Job drawing, mm, ordinate dimensions from the low corner. One solid piece. A direction names the side the tool comes from. Round coordinates to 2 decimals unless told otherwise and drop trailing zeros. Loops run counter-clockwise (first coordinate to the right, second up) from the corner with the lowest first, then second, coordinate; pieces in that order, holes last.
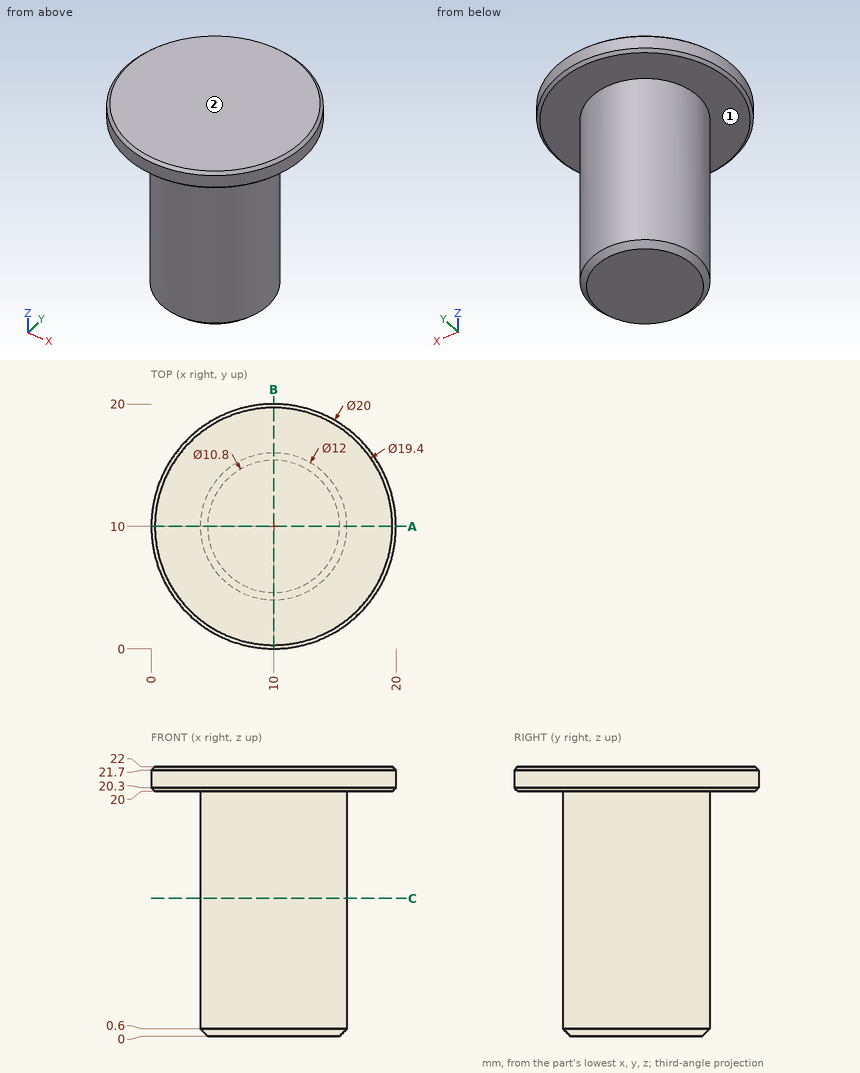
Item 1: Cut at C-C, the plane z = 11.25. Give the cut face in (x, y).
Answers follow:
outline: circle Ø12 at (10, 10)
Item 2: 3-axis set-ups, long thin cutter, end or side, ignore diameter. For the marked faces 1 and 2: which of +Z, -Z, +X, -X, +Y, -Y reach the whole face in a straight line?
Answers follow:
face 1: -Z
face 2: +Z, +X, -X, +Y, -Y
Item 3: Flat gauge pins, fed straight in: P1, Ø2, axis at y = 12, z = 12, coming from the -X side; P2, Ø6, axis at x = 17, z = 18.5, coming from the -Y side; P3, Ø2, axis at y = 10.5, z = 14, coming from the -X side. Where does each tip first touch, or does it go through?
Answers follow:
P1: stops at x = 4.08
P2: stops at y = 1.12
P3: stops at x = 4
Item 4: Probe line 1 (Z direction, x = 2, y = 8); line 2 (Y direction, x = 9.5, z = 21.25); line 3 (X direction, y = 10.5, z = 10.75). List the from-to ranges inside material, lowest first.
Answers follow:
line 1: z = 20 to 22
line 2: y = 0.01 to 19.99
line 3: x = 4.02 to 15.98
Item 5: Cut at A-A, the plane y = 10. Give the cut face in (x, z), plus the area to 3 significant figures.
Answers follow:
outline: (0, 20.3) - (0.3, 20) - (4, 20) - (4, 0.6) - (4.6, 0) - (15.4, 0) - (16, 0.6) - (16, 20) - (19.7, 20) - (20, 20.3) - (20, 21.7) - (19.7, 22) - (0.3, 22) - (0, 21.7) - close
area: 279 mm2
